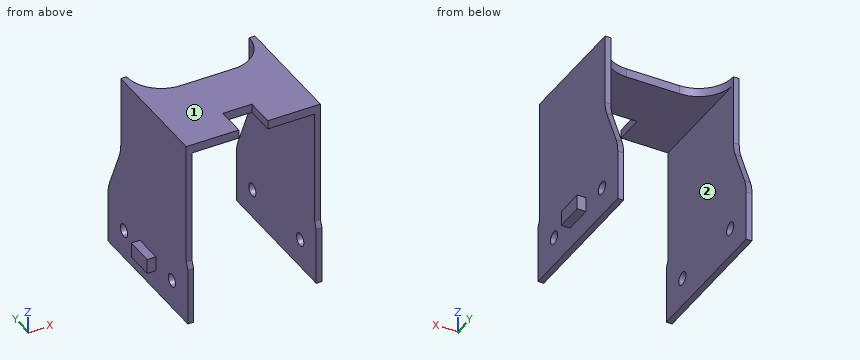
from build123d import *

# Parameters (mm, degrees)
SKETCH_1_W                   = 2
SKETCH_1_H                   = 10
EXTRUDE_1_DEPTH              = 62
EXTRUDE_1_2_DEPTH            = 62
SKETCH_2_W                   = 46.4
SKETCH_2_H                   = 10
EXTRUDE_2_DEPTH              = 3
SKETCH_3_W                   = 2
SKETCH_3_H                   = 20
EXTRUDE_3_DEPTH              = 20
EXTRUDE_4_DEPTH              = 2
MIRROR_3_COPY_1_SKETCH_W     = 2
MIRROR_3_COPY_1_SKETCH_H     = 20
MIRROR_3_COPY_1_DEPTH        = 20
MIRROR_3_COPY_2_DEPTH        = 2
MIRROR_3_COPY_3_SKETCH_W     = 2
MIRROR_3_COPY_3_SKETCH_H     = 20
MIRROR_3_COPY_3_DEPTH        = 20
EXTRUDE_5_DEPTH              = 9
HOLE_WIZARD_M4_1_D           = 4.5
HOLE_WIZARD_M4_1_CSINK_D     = 4.55
HOLE_WIZARD_M4_1_CSINK_ANGLE = 90
SKETCH_10_W                  = 5.1
SKETCH_10_H                  = 10
EXTRUDE_6_DEPTH              = 3
EXTRUDE_7_DEPTH              = 10
EXTRUDE_8_REACH              = 76.407
SKETCH_12_W                  = 2
SKETCH_12_H                  = 22
SKETCH_13_W                  = 10
SKETCH_13_H                  = 10
CUT_EXTRUDE_1_DEPTH          = 10
FILLET_1_R                   = 12
FILLET_2_R                   = 12


with BuildPart() as part:
    # Sketch 1 → Extrude 1 (new body)
    with BuildSketch(Plane.XY):
        with Locations((-22.2, 0)):
            Rectangle(SKETCH_1_W, SKETCH_1_H)
    extrude(amount=EXTRUDE_1_DEPTH)



with BuildPart() as body_2:
    # Sketch 1 → Extrude 1 2 (new body)
    with BuildSketch(Plane.XY):
        with Locations((22.2, 0)):
            Rectangle(SKETCH_1_W, SKETCH_1_H)
    extrude(amount=EXTRUDE_1_2_DEPTH)


with BuildPart() as part_1:
    add(part.part)

    add(body_2.part)  # Extrude 2 merges body 2
    # Sketch 2 → Extrude 2 (add)
    with BuildSketch(Plane.XY.offset(62)):
        Rectangle(SKETCH_2_W, SKETCH_2_H)
    extrude(amount=EXTRUDE_2_DEPTH)

    # Sketch 3 → Extrude 3 (add)
    with BuildSketch(Plane(origin=(0, 5, 0), x_dir=(1, 0, 0), z_dir=(0, 1, 0))):
        with Locations((-22.2, -10)):
            Rectangle(SKETCH_3_W, SKETCH_3_H)
        with Locations((22.2, -10)):
            Rectangle(SKETCH_3_W, SKETCH_3_H)
    extrude_3 = extrude(amount=EXTRUDE_3_DEPTH)

    # Sketch 4 → Extrude 4 (add)
    with BuildSketch(Plane.ZY.offset(-21.2)):
        Polygon((20, 25), (20, 5), (65, 5), align=None)
    extrude_4 = extrude(amount=-EXTRUDE_4_DEPTH)

    # Mirror 1: Extrude 3, Extrude 4 across plane
    add(extrude_3.mirror(Plane.ZX))
    add(extrude_4.mirror(Plane.ZX))

    # Mirror 3: Extrude 4 across plane
    add(extrude_4.mirror(Plane.ZY))

    # Mirror 3 copy 1 sketch → Mirror 3 copy 1 (add)
    with BuildSketch(Plane(origin=(0, -5, 0), x_dir=(-1, 0, 0), z_dir=(0, -1, 0))):
        with Locations((-22.2, -10)):
            Rectangle(MIRROR_3_COPY_1_SKETCH_W, MIRROR_3_COPY_1_SKETCH_H)
        with Locations((22.2, -10)):
            Rectangle(MIRROR_3_COPY_1_SKETCH_W, MIRROR_3_COPY_1_SKETCH_H)
    extrude(amount=MIRROR_3_COPY_1_DEPTH)

    # Mirror 3 copy 2 sketch → Mirror 3 copy 2 (add)
    with BuildSketch(Plane(origin=(-21.2, 0, 0), x_dir=(0, 0, 1), z_dir=(1, 0, 0))):
        Polygon((20, 25), (20, 5), (65, 5), align=None)
    extrude(amount=-MIRROR_3_COPY_2_DEPTH)

    # Mirror 3 copy 3 sketch → Mirror 3 copy 3 (add)
    with BuildSketch(Plane(origin=(0, 5, 0), x_dir=(-1, 0, 0), z_dir=(0, 1, 0))):
        with Locations((-22.2, 10)):
            Rectangle(MIRROR_3_COPY_3_SKETCH_W, MIRROR_3_COPY_3_SKETCH_H)
        with Locations((22.2, 10)):
            Rectangle(MIRROR_3_COPY_3_SKETCH_W, MIRROR_3_COPY_3_SKETCH_H)
    extrude(amount=MIRROR_3_COPY_3_DEPTH)

    # Sketch 6 → Extrude 5 (add)
    with BuildSketch(Plane.XZ.offset(5)):
        Polygon((-23.2, 65), (-23.2, 44.637351208), (-21.2, 44.637351208), (-21.2, 62), (21.2, 62), (21.2, 45), (23.2, 45), (23.2, 65), align=None)
    extrude(amount=EXTRUDE_5_DEPTH)

    # Hole Wizard M4 _ _1 (through all)
    with Locations(Plane(origin=(23.2, 0, 0), x_dir=(0, 0, -1), z_dir=(1, 0, 0))):
        with Locations((-10, -15), (-10, 15)):
            CounterSinkHole(HOLE_WIZARD_M4_1_D / 2, HOLE_WIZARD_M4_1_CSINK_D / 2, counter_sink_angle=HOLE_WIZARD_M4_1_CSINK_ANGLE)

    # Sketch 10 → Extrude 6 (add)
    with BuildSketch(Plane(origin=(23.2, 0, 0), x_dir=(0, 0, -1), z_dir=(1, 0, 0))):
        with Locations((-10, 0)):
            Rectangle(SKETCH_10_W, SKETCH_10_H)
    extrude_6 = extrude(amount=EXTRUDE_6_DEPTH)

    # Mirror 4: Extrude 6 across plane
    add(extrude_6.mirror(Plane.ZY))

    # Sketch 11 → Extrude 7 (add)
    with BuildSketch(Plane.XZ.offset(14)):
        Polygon((-23.2, 15), (-21.2, 15), (-21.2, 62), (21.2, 62), (21.2, 15), (23.2, 15), (23.2, 65), (-23.2, 65), align=None)
    extrude(amount=EXTRUDE_7_DEPTH)

    # Sketch 12 → Extrude 8 (add, up to next)
    with BuildSketch(Plane.XY.offset(65), mode=Mode.PRIVATE) as extrude_8_sk1:
        with Locations((-22.2, 6)):
            Rectangle(SKETCH_12_W, SKETCH_12_H)
    extrude_8_tool1 = extrude(extrude_8_sk1.sketch, amount=-EXTRUDE_8_REACH, mode=Mode.PRIVATE) - part_1.part
    # Sketch 12 → Extrude 8 (add, up to next)
    with BuildSketch(Plane.XY.offset(65), mode=Mode.PRIVATE) as extrude_8_sk2:
        with Locations((22.2, 6)):
            Rectangle(SKETCH_12_W, SKETCH_12_H)
    extrude_8_tool2 = extrude(extrude_8_sk2.sketch, amount=-EXTRUDE_8_REACH, mode=Mode.PRIVATE) - part_1.part
    add(extrude_8_tool1.solids().sort_by_distance((-22.2, 6, 65))[0])
    add(extrude_8_tool2.solids().sort_by_distance((22.2, 6, 65))[0])

    # Sketch 13 → Cut-Extrude 1 (cut)
    with BuildSketch(Plane.XY.offset(65)):
        with Locations((0, -19)):
            Rectangle(SKETCH_13_W, SKETCH_13_H)
    extrude(amount=-CUT_EXTRUDE_1_DEPTH, mode=Mode.SUBTRACT)

    # Fillet 1
    fillet_1_edges = [part_1.edges().sort_by_distance(p)[0] for p in [
        (21.2, 5, 63.5),
        (-21.2, 5, 63.5),
    ]]
    fillet(fillet_1_edges, radius=FILLET_1_R - 0.0001)  # a hair under: the kernel refuses the full size

    # Fillet 2
    fillet_2_edges = [part_1.edges().sort_by_distance(p)[0] for p in [
        (-22.2, 17, 38),
        (22.2, 17, 38),
        (-22.2, 25, 20),
        (22.2, 25, 20),
    ]]
    fillet(fillet_2_edges, radius=FILLET_2_R)


solid = part_1.part
Verification items for the finished model (mm, model axes). Face numbers are marked on the shaded views. A direction names the side the tool comes from. Coordinates: 2 decimals unless noted, no trailing zeros. Order: outer loops, then holes, each group sorted by start corner. A loop starts at its lowest first (then second) coordinate and runs counter-clockwise, first axis right, second up.
Item 1: Section check A-A, the plane z = 15.5. Enter the section's corners in (x, y).
Filled in:
outline: (-23.2, -25) - (-21.2, -25) - (-21.2, 25) - (-23.2, 25) - close; (21.2, -25) - (23.2, -25) - (23.2, 25) - (21.2, 25) - close
Item 2: Section check D-D, the plane x = -1. Enter the section's corners in (y, z).
Filled in:
outline: (-14, 62) - (5, 62) - (5, 65) - (-14, 65) - close
Item 3: Section check B-B, the plane y = -15. Enter the section's corners in (x, z) (3 decimals).
Filled in:
outline: (-23.2, 0) - (-21.2, 0) - (-21.2, 7.75) - (-23.2, 7.75) - close; (-23.2, 12.25) - (-21.2, 12.25) - (-21.2, 62) - (-5, 62) - (-5, 65) - (-23.2, 65) - close; (5, 62) - (21.2, 62) - (21.2, 12.25) - (23.175, 12.25) - (23.2, 12.275) - (23.2, 65) - (5, 65) - close; (21.2, 0) - (23.2, 0) - (23.2, 7.725) - (23.175, 7.75) - (21.2, 7.75) - close
Item 4: Access from +Z, -Z, +X, -X, +Y, -Y to the whole of each face (thin tool, end or side, straight path). Record for the marked faces 1 and 2.
Filled in:
face 1: +Z, +X, -X, +Y, -Y
face 2: -Z, +Y, -Y
Item 5: Material ranges on L1, parallel to Y at x = -22.6, z = 10; L2, parallel to X at y = -6.5, z = 23; L3, parallel to Z at x = 22, y = -15, recorded low to high.
Filled in:
L1: y = -25 to -17.25, -12.75 to 12.75, 17.25 to 25
L2: x = -23.2 to -21.2, 21.2 to 23.2
L3: z = 0 to 7.75, 12.25 to 65
Item 6: Section check C-C, the plane z = 43.5. Enter the section's corners in (x, y), then the cut area to 3 significant figures.
Filled in:
outline: (-23.2, -24) - (-21.2, -24) - (-21.2, 17) - (-23.2, 17) - close; (21.2, -24) - (23.2, -24) - (23.2, 17) - (21.2, 17) - close
area: 164 mm2
Item 7: Depth check by flat-ended pin: pin 1 (12.5 mm diameter, centred on x = 3.5, y = -5, fed in from -Z); pin 2 (4 mm diameter, centred on y = 3, z = 54, fed in from +X); pin 3 (0.9 mm diameter, centred on x = -2, z = 64, fed in from +Y); pin 4 (3.5 mm diameter, centred on x = 24, y = 2, fed in from -Z). Enter the tip coordinate at first touch or a pass-through.
Filled in:
pin 1: stops at z = 62
pin 2: stops at x = 23.2
pin 3: stops at y = 5
pin 4: stops at z = 0
